Source: CAD feature listing. Evaluate the final solid. Frame: model axes, mm. A direction names the side the tool comes from. Give positions to 0.01 mm unless a question says otherwise; leave off trailing zeros. Write each loop counter-clockwise with the first axis right and the second up, starting at its lowest first coordinate (ties: lowest second). Pieces come first, ordered by that corner, then holes. Notation, with made-up numbers: (74, 59.25) -> (100, 59.25) arc R31 cw to (100, 86.25) -> close; hole circle Ø11 at (-3.75, 21.25). An arc over 180 degrees is marked (long way). Answer as a JSON object with one key per item and string values. Group by question number.
Item 1: Section query D-D on x = -3. Return the cut outline in (y, z).
Item 2: Section query B-B on z = -11. Return the cut outline in (x, y).
Item 3: Section query C-C on y = -4.25. Return the cut outline in (x, z).
Item 4: Access query for faces 1 (the face through (12, -1, 26.65)), 2 (the face through (0, -4, 28.65)), 3 (the face through (29, -1, -6)), 4 (the face through (6, -1, -29)). Directions: +Z, -Z, +X, -X, +Y, -Y. A direction counts if a zero-diameter tool reaches every point of the face in a straight line with its end or side. Return the directions, or none.
Item 5: Pull-direction query (Z, two-part tool) for faces 5 (the face through (0, -3, -30.15)), 6 (the face through (-29, -1, -6)), 7 (the face through (-23, 0, -23)); classes: pulls with the +Z half, pulls with the -Z half, needs draft (parallel to the pull), parting line crosses it, or undercut.
Item 6: First-contact query: pin 1 Ø1.2 at (x, z) = (-29.5, -1) entering from +Y; pin 2 Ø12 at (x, z) = (-20, -2.5) entering from -Y. Flat tips, straight axial feed; report the tip coordinate or a pass-through.
Item 7: Section query A-A on x = 10. Return the cut outline in (y, z).
Item 8: Ray query, probe 1 along X at (y, z) = (-3.5, 2); probe 2 along Z at (x, y) = (26, -1.25). Return the intervals inside material, ascending. Write a range as from..to.
from build123d import *

# Parameters (mm, degrees)
F0_W     = 57.3
F0_H     = 57.3
F1_DEPTH = 1.5
F2_W     = 57.3
F2_H     = 57.3
F3_DEPTH = 7
F5_DEPTH = 2.5


with BuildPart() as f1:
    # F0 (on Front) → F1 (new body)
    with BuildSketch(Plane.XZ):
        Rectangle(F0_W, F0_H)
        Polygon((-18.164719, 26.65), (18.164719, 26.65), (26.65, 18.164719), (26.65, -18.164719), (18.164719, -26.65), (-18.164719, -26.65), (-26.65, -18.164719), (-26.65, 18.164719), align=None, mode=Mode.SUBTRACT)
    extrude(amount=F1_DEPTH)

    # F2 (on Front) → F3 (join)
    with BuildSketch(Plane.XZ):
        Polygon((28.65, 30.15), (-28.65, 30.15), (-30.15, 30.15), (-30.15, 28.65), (-30.15, -28.65), (-30.15, -30.15), (-28.65, -30.15), (28.65, -30.15), (30.15, -30.15), (30.15, -28.65), (30.15, 28.65), (30.15, 30.15), align=None)
        Rectangle(F2_W, F2_H, mode=Mode.SUBTRACT)
    extrude(amount=F3_DEPTH)

    # F4 (on Front) → F5 (cut)
    with BuildSketch(Plane.XZ):
        Polygon((25.578076, 6), (25.578076, 0), (25.578076, -6), (33.948865, -6), (33.948865, 6), align=None)
        Polygon((-6, 33.948865), (-6, 25.578076), (0, 25.578076), (6, 25.578076), (6, 33.948865), align=None)
        Polygon((-33.948865, -6), (-25.578076, -6), (-25.578076, 0), (-25.578076, 6), (-33.948865, 6), align=None)
        Polygon((6, -33.948865), (6, -25.578076), (0, -25.578076), (-6, -25.578076), (-6, -33.948865), align=None)
    extrude(amount=F5_DEPTH, mode=Mode.SUBTRACT)


solid = f1.part
Worked answers:
{
 "1": {"outline": "(-7, -30.15) -> (-2.5, -30.15) -> (-2.5, -28.65) -> (-7, -28.65) -> close; (-7, 28.65) -> (-2.5, 28.65) -> (-2.5, 30.15) -> (-7, 30.15) -> close"},
 "2": {"outline": "(-30.15, -7) -> (-28.65, -7) -> (-28.65, -1.5) -> (-26.65, -1.5) -> (-26.65, 0) -> (-30.15, 0) -> close; (26.65, -1.5) -> (28.65, -1.5) -> (28.65, -7) -> (30.15, -7) -> (30.15, 0) -> (26.65, 0) -> close"},
 "3": {"outline": "(-30.15, -30.15) -> (30.15, -30.15) -> (30.15, 30.15) -> (-30.15, 30.15) -> close; hole (-28.65, -28.65) -> (28.65, -28.65) -> (28.65, 28.65) -> (-28.65, 28.65) -> close"},
 "4": {"face 1": "+Y, -Y", "face 2": "-Y", "face 3": "+X, -X, +Y", "face 4": "+Z, -Z, +Y"},
 "5": {"face 5": "pulls with the -Z half", "face 6": "undercut", "face 7": "needs draft"},
 "6": {"pin 1": "y = -2.5", "pin 2": "through"},
 "7": {"outline": "(-7, -30.15) -> (0, -30.15) -> (0, -26.65) -> (-1.5, -26.65) -> (-1.5, -28.65) -> (-7, -28.65) -> close; (-7, 28.65) -> (-1.5, 28.65) -> (-1.5, 26.65) -> (0, 26.65) -> (0, 30.15) -> (-7, 30.15) -> close"},
 "8": {"probe 1": "-30.15..-28.65, 28.65..30.15", "probe 2": "-30.15..-18.81, 18.81..30.15"}
}
